```python
from build123d import *

# Parameters (mm, degrees)
F0_R      = 47.625
F1_DEPTH  = 38.1
F1_TAPER  = -10
F2_R      = 46.355
F3_DEPTH  = 38.1
F3_TAPER  = -10
F4_DEPTH  = 3.175
F7_SIZE   = 2.032
F9_DEPTH  = 12.7
F10_R     = 8.128
F11_DEPTH = 25.4
F11_TAPER = -3


with BuildPart() as f1:
    # F0 (on Top) → F1 (new body)
    with BuildSketch(Plane.XY):
        Circle(F0_R)
    extrude(amount=F1_DEPTH, taper=F1_TAPER)

    # F2 (on Top) → F3 (cut)
    with BuildSketch(Plane.XY):
        Circle(F2_R)
    extrude(amount=F3_DEPTH, taper=F3_TAPER, mode=Mode.SUBTRACT)

    # F0 (on Top) → F4 (join)
    with BuildSketch(Plane.XY):
        Circle(F0_R)
    extrude(amount=-F4_DEPTH)

    # F5 (on Front) → F6 (revolve)
    with BuildSketch(Plane.XZ):
        Polygon((0, 46.8748211861), (0, 0), (3.5949361045, 0), (2.1285163239, 46.8748211861), align=None)
    revolve(axis=Axis((0, 0, 0), (0, 0, 1)))

    # F7
    f7_edges = [f1.edges().sort_by_distance(p)[0] for p in [
        (-2.128516, 0, 46.874821),
    ]]
    chamfer(f7_edges, length=F7_SIZE)

    # F8 (on face) → F9 (join)
    with BuildSketch(Plane.XY.offset(38.1)):
        with BuildLine():
            Line((69.9530094796, 41.4682495986), (33.1230094796, 41.4682495986))
            ThreePointArc((33.1230094796, 41.4682495986), (52.9801221963, 0.348952149), (33.6663710675, -41.0283431411))
            Line((33.6663710675, -41.0283431411), (69.9530094796, -41.0283431411))
            Line((69.9530094796, -41.0283431411), (69.9530094796, 41.4682495986))
        make_face()
    extrude(amount=-F9_DEPTH)

    # F10 (on face) → F11 (cut)
    with BuildSketch(Plane(origin=(0, 0, 25.4), x_dir=(1, 0, 0), z_dir=(0, 0, -1))):
        with Locations((57.9903379162, -29.164113198)):
            Circle(F10_R)
    extrude(amount=-F11_DEPTH, taper=F11_TAPER, mode=Mode.SUBTRACT)


solid = f1.part
```
The model under review builds one solid part; all positions refer to its coordinate system, in mm. A direction names the side the tool comes from. Round coordinates to 2 decimals unless told otherwise and drop trailing zeros. Order: outer loops, then holes, each group sorted by start corner. A loop starts at its lowest first (then second) coordinate and runs counter-clockwise, first axis right, second up. Notation, with made-up numbers: (76.25, -19.75) -> (86.25, -19.75) arc R18 cw to (86.25, -10.75) -> close; hole circle Ø1 at (-11, 54.5). An arc over 180 degrees is marked (long way). One line per item, written item: value. Start each with the question number.
Q1. Mouldability with a two-part tool opening along X and no side actions: class faces 1 (the face through (-37.794, -28.979, -1.565)), 2 (the face through (52.97, 1.01, 37.9)), 3 (the face through (-1, -10, 0)), 4 (the face through (52, 41.468, 32)) as released by +X, released by -X, zero draft, split by the parting line, or undercut.
Q2. Take a section at A-A (z = 9.5). Write out the cut boundary in (x, y), and give its area (3 significant figures).
Q3. Wall thickness on line 1 (X direction, y = -28, z = 27) (3 decimals); line 2 (Y direction, x = 3, z = 8.5); line 3 (Z direction, x = -6.5, y = -39) (3 decimals): over which ranges is each line inside the solid? List them lowest first.
Q4. Machinability: for faces 5 (the face through (-1, 1, -3.175)), 6 (the face through (59, 1, 25.4)), 7 (the face through (2.75, 0.87, 22.74)), which of the approach directions +Z, -Z, +X, -X, +Y, -Y give a long, thin tool a straight path to every point of the face, cutting with its end or side? Answer none if there is none.
Q5. Clearance check with flat-ended pins moving along their axes: pin 1 Ø6 at (x, z) = (43, 21) entering from +Y; pin 2 Ø5 at (x, y) = (-11.5, -8.5) entering from +Z; pin 3 Ø10 at (x, z) = (26.5, 16.5) entering from -Y. State where each tip first meets the part, or that it passes through.
Reported:
1. face 1: split by the parting line
1. face 2: undercut
1. face 3: undercut
1. face 4: zero draft
2. outline: circle Ø98.6 at (0, 0); circle Ø6.6 at (0, 0); hole circle Ø96.06 at (0, 0)
2. area: 422 mm2
3. line 1: x = -44.275 to -42.765, 42.765 to 44.275, 45.023 to 69.953
3. line 2: y = -49.03 to -47.76, -1.44 to 1.44, 47.76 to 49.03
3. line 3: z = -3.175 to 0
4. face 5: -Z, +X, -X, +Y, -Y
4. face 6: -Z, +X
4. face 7: +Z
5. pin 1: stops at y = 32.26
5. pin 2: stops at z = 0
5. pin 3: stops at y = -45.93
